Part print with two shaded views. Sizes in mm from the minimum x, y, z corner. Give positions to 0.01 mm unless a question says otherwise; leave off trailing zeros. Order: outer loops, then holes, each group sorted by start corner. A loop starts at its lowest first (then second) coordinate and runs counter-clockwise, first axis right, second up. Notation, with made-up numbers: M -7.5,78.25 L 15.5,78.25 A18 cw 15.5,91.25 Z; hole C 31.25,46.25 d10. An arc over 180 degrees is marked long. Return JSON: item names as keys, results as strings. Group by question number.
1. Slice it at A-A on z = 3.7. List the corners of the cut face in (x, y).
2. Wall check: probe 1 along X at (y, z) = (6, 2.7); probe 2 along Z at (x, y) = (3.35, 2) (1 decimal); probe 3 along X at (y, z) = (6, 3.5). Give the ranges that are in metal, low to high. Write a range as [from, to].
3. Slice it at C-C on y = 2.25. List the corners of the cut face in (x, z), then the cut area to 3 significant figures.
4. Slice it at D-D on z = 0.85. List the corners of the cut face in (x, y).
5. Slice it at B-B on x = 2.5. List the corners of the cut face in (y, z) (1 decimal).
6. Two-plate mould, pull along Z, no slides. Class the marked faces 1, 2, 3 and 4: released by +Z, released by -Z, zero draft, split by the parting line, or undercut.
7. Pin check, flat tips, straight feed: pin 1 (1.5 mm diameter, centred on x = 1.5, y = 4, fed in from +Z); pin 2 (1 mm diameter, centred on x = 1, z = 1.5, fed in from -Y); pin 3 (1.5 mm diameter, centred on x = 2.3, z = 2.66, fed in from -Y). Stop position of each tip, or through.
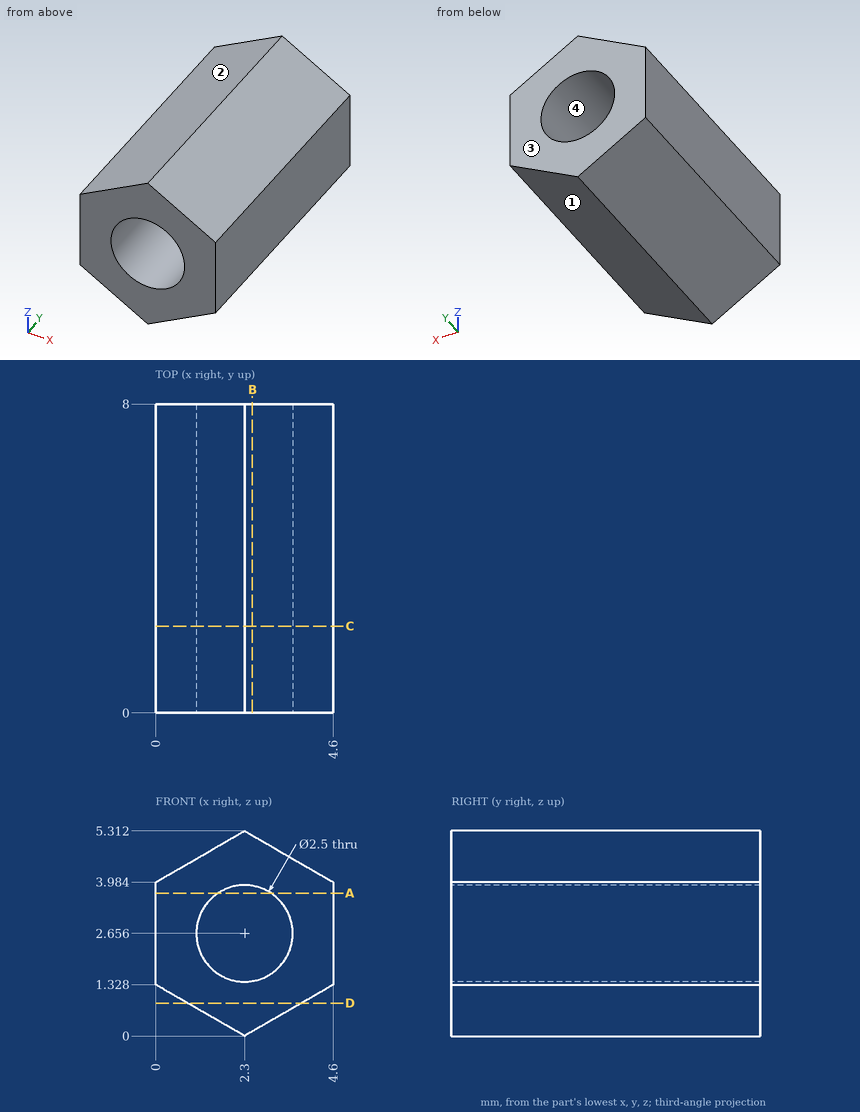
Result:
{
 "1": {"outline": "M 0,0 L 1.61,0 L 1.61,8 L 0,8 Z; M 2.99,0 L 4.6,0 L 4.6,8 L 2.99,8 Z"},
 "2": {"probe 1": "x = [0, 1.05], [3.55, 4.6]", "probe 2": "z = [0.6, 2], [3.3, 4.7]", "probe 3": "x = [0, 1.38], [3.22, 4.6]"},
 "3": {"outline": "M 0,1.33 L 2.3,0 L 4.6,1.33 L 4.6,3.98 L 2.3,5.31 L 0,3.98 Z; hole C 2.3,2.66 d2.5", "area": "13.4 mm2"},
 "4": {"outline": "M 0.83,0 L 3.77,0 L 3.77,8 L 0.83,8 Z"},
 "5": {"outline": "M 0,0.1 L 8,0.1 L 8,1.4 L 0,1.4 Z; M 0,3.9 L 8,3.9 L 8,5.2 L 0,5.2 Z"},
 "6": {"face 1": "released by -Z", "face 2": "released by +Z", "face 3": "zero draft", "face 4": "undercut"},
 "7": {"pin 1": "stops at z = 5.28", "pin 2": "stops at y = 0", "pin 3": "passes through"}
}
